Verification items for the finished model (mm, model axes). A direction names the side the tool comes from. Round coordinates to 2 decimals unless told otherwise and drop trailing zeros. Write each loop counter-clockwise with the first axis right and the second up, starting at its lowest first coordinate (ties: lowest second). Pieces come first, ordered by that corner, then holes. Notation, with made-up numbers: (-4, 9.5) - (51, 9.5) arc R34 cw to (51, 39.5) - close; hole circle Ø1 at (11.5, 64). An arc over 180 degrees is marked (long way). Answer as a JSON object with one key per item and string values.
Autodesk Inventor part; units mm, degrees
ref_plane "Work Plane7" through (30.1625, -2.4255, 381.254) normal (0.258819, 0, 0.9659258) x (0, 1, 0)
ref_plane "YZ Plane" through (0, 0, 0) normal (1, 0, 0) x (0, 1, 0)
ref_plane "XZ Plane" through (0, 0, 0) normal (0, 1, 0) x (-1, 0, 0)
sketch "Sketch1" plane through (0, 0, 0) normal (0, 0, 1) x (1, 0, 0)
  circle A0 centre (0, 0) radius 30.1625
  circle A1 centre (0, 0) radius 26.2509
  dimension "d0" = 60.325
  dimension "d2" = 3.9116
extrude "Extrusion1" add sketch "Sketch1" along normal blind 381
sketch "Sketch16" plane through (0, 0, 381) normal (0, 0, 1) x (1, 0, 0)
  circle A0 centre (0, 0) radius 30.1625
  line L0 (27.5395, -2.4255) -> (30.1625, -2.4255)
  line L1 (30.1625, -2.4255) -> (30.1625, 0)
  line L2 (30.1625, 0) -> (27.5395, 0)
  line L3 (27.5395, 0) -> (27.5395, -2.4255)
extrude "Extrusion9" add sketch "Sketch16" along normal blind 0.254 contours L1 L0 A0 | A0 L0 L3 L2 picked at (28.3994, -1.3478)
ref_plane "Work Plane7" through (30.1625, -2.4255, 381.254) normal (0.258819, 0, 0.9659258) x (0, 1, 0)
sketch "Sketch17" plane through (30.1625, -2.4255, 381.254) normal (0.258819, 0, 0.9659258) x (0, 1, 0)
  circle A0 centre (2.4255, 29.9579) radius 30.1625
  circle A1 centre (2.4255, 29.9579) radius 26.2509
  point P0 (2.4255, -69.5411)
  dimension "d54" = 60.325
  dimension "d55" = 3.9116
extrude "Extrusion10" add sketch "Sketch17" along normal blind 25.4 draft 0.2 and the other way blind 15.24
properties part number "2r2scs" material "PVC-Piping"
1. Mould release check, pull along X, two halves, no side actions. Record for faces 4 (the face through (-4.21, 28.81, 403.8)), 5 (the face through (-13.98, -13.59, 419.38)), 6 (the face through (23.628, -0.123, 367.227)): released by +X, released by -X, zero draft, split by the parting line, or undercut.
Completed:
{"face 4": "split by the parting line", "face 5": "released by +X", "face 6": "undercut"}
2. Access from +Z, -Z, +X, -X, +Y, -Y to the whole of each face (thin tool, end or side, straight path). Record for faces 1 (the face through (-30.133, -1.326, 187.833)), 2 (the face through (-9, 25, 0)), 3 (the face through (-26.4, 2.1, 381)).
Completed:
{"face 1": "-Z", "face 2": "-Z, +X, -X, +Y, -Y", "face 3": "none"}
3. Cross-section at A-A (z = 171). Record the boundary of the cut face in (x, y) (1 decimal), plus the area to 3 significant figures.
Completed:
{"outline": "circle Ø60.3 at (0, 0); hole circle Ø52.5 at (0, 0)", "area": "693 mm^2"}
4. Go/stop test with flat-tipped pins: pin 1 (4 mm diameter, centred on y = -0.5, z = 248, fed in from -X); pin 2 (6 mm diameter, centred on y = -20.5, z = 152, fed in from -X); pin 3 (6 mm diameter, centred on x = -3.5, z = 159, fed in from -Y). Record where each tip stops, or that it passes through.
Completed:
{"pin 1": "stops at x = -30.16", "pin 2": "stops at x = -24.57", "pin 3": "stops at y = -30.16"}
5. Material ranges on probe 1 along X at (y, z) = (0, 293), recorded low to high. Write a range as from..to.
Completed:
{"probe 1": "x = -30.16..-26.25, 26.25..30.16"}
